from build123d import *

# Parameters (mm, degrees)
BOSS_EXTRUDE1_DEPTH      = 37.1475
BOSS_EXTRUDE1_DEPTH_BACK = 37.1475
SKETCH3_R                = 4.7625


with BuildPart() as part:
    # Sketch3 → Boss-Extrude1 (new, two sides: drawn at the far end of the back side and taken through both)
    with BuildSketch(Plane.XY.offset(-BOSS_EXTRUDE1_DEPTH_BACK)):
        Circle(SKETCH3_R)
    extrude(amount=BOSS_EXTRUDE1_DEPTH + BOSS_EXTRUDE1_DEPTH_BACK)

    # Sketch6 → Tap Drill for M5x0.8 Tap1 (revolve, cut)
    with BuildSketch(Plane(origin=(0, 0, 37.1475), x_dir=(0, -1, 0), z_dir=(1, 0, 0))):
        Polygon((0, 0), (0, 13.9618073), (2.1, 12.7), (2.1, 0), align=None)
    tap_drill_for_m5x0_8_tap1 = revolve(axis=Axis((0, 0, 43.4975), (0, 0, -1)), mode=Mode.SUBTRACT)

    # Mirror1: Tap Drill for M5x0.8 Tap1 across plane
    add(tap_drill_for_m5x0_8_tap1.mirror(Plane.XY), mode=Mode.SUBTRACT)


solid = part.part
Here's how the part is built. I have some questions about the finished solid (model axes, mm). A direction names the side the tool comes from. Coordinates: 2 decimals unless noted, no trailing zeros. Write each loop counter-clockwise with the first axis right and the second up, starting at its lowest first coordinate (ties: lowest second). Pieces come first, ordered by that corner, then holes.
Item 1: On a 3-axis mill with a long thin cutter (end or side, diameter ignored), from which of +Z, -Z, +X, -X, +Y, -Y can I reach the whole of each face in a straight line? I mean faces 4 (the conical face through (0.356, 0.079, -23.405)), 5 (the cylindrical face through (-0.631, -2.003, 30.886)). Say none if no direction works.
Item 2: If I drill on line 1 (Y direction, x = 0, z = -30); line 2 (Y direction, x = -0.25, z = 12); line 3 (Y direction, x = 1.5, z = 25.5), over which ranges is the centre line in solid material (lowest first)?
Item 3: I want a section at A-A on z = -32. Write out the boundary of the cut face in (x, y) (1 decimal), and give its area (3 significant figures).
Item 4: If we mould it in two halves opening along Y, with no side actions, what happens to faces 1 (the cylindrical face through (-3.78, -2.9, -0.52)), 2 (the flat face through (2.05, -0.99, -37.148)), 3 (the cylindrical face through (-0.631, -2.003, -30.886))? For each: +Y half, -Y half, draft (parallel to the pull), parting line (faces both ways), or undercut.
Item 5: I want a section at C-C on x = 3. Write out the boundary of the cut face in (y, z), and give its area (3 significant figures).
Item 6: Will these pins go through, and if not, where does the flat tip stop? pin 1 (5 mm diameter, centred on x = -1.5, y = -0.5, fed in from -Z); pin 2 (2.5 mm diameter, centred on x = 0, y = 0, fed in from +Z); pin 3 (1.5 mm diameter, centred on x = 2, z = -27.5, fed in from -Y); pin 4 (3 mm diameter, centred on x = -2.5, z = 4, fed in from -Y).
Item 7: I want a section at B-B on z = 12.5. Write out the boundary of the cut face in (x, y) (1 decimal).
Findings below:
1. face 4: -Z
1. face 5: +Z
2. line 1: y = -4.76 to -2.1, 2.1 to 4.76
2. line 2: y = -4.76 to 4.76
2. line 3: y = -4.52 to -1.47, 1.47 to 4.52
3. outline: circle Ø9.5 at (0, 0); hole circle Ø4.2 at (0, 0)
3. area: 57.4 mm2
4. face 1: parting line
4. face 2: draft
4. face 3: undercut
5. outline: (-3.7, -37.15) - (3.7, -37.15) - (3.7, 37.15) - (-3.7, 37.15) - close
5. area: 550 mm2
6. pin 1: stops at z = -37.15
6. pin 2: stops at z = 23.94
6. pin 3: stops at y = -4.6
6. pin 4: stops at y = -4.66
7. outline: circle Ø9.5 at (0, 0)
